CAD build for the part. Positions are in the model's coordinates, mm. A direction names the side the tool comes from. Coordinates: 2 decimals unless noted, no trailing zeros. Loops run counter-clockwise (first coordinate to the right, second up) from the corner with the lowest first, then second, coordinate; pieces in that order, holes last. Notation, with made-up numbers: (-19.5, 66) -> (21.5, 66) arc R9 ccw to (21.5, 82) -> close; hole circle Ø5 at (30, 49.5). An arc over 180 degrees is marked (long way). Answer as a JSON object with one key per item and string values. Group by question number.
from build123d import *

# Parameters (mm, degrees)
SKETCH1_W                                  = 254
SKETCH1_H                                  = 203.2
BOSS_EXTRUDE1_DEPTH                        = 6.35
SKETCH2_W                                  = 6.35
SKETCH2_H                                  = 190.5
BOSS_EXTRUDE2_DEPTH                        = 63.5
SKETCH3_W                                  = 6.35
SKETCH3_H                                  = 40.64
CUT_EXTRUDE1_DEPTH                         = 63.5
SKETCH4_W                                  = 50.8
SKETCH4_H                                  = 40.64
CUT_EXTRUDE2_DEPTH                         = 3.175
SKETCH5_W                                  = 31.75
SKETCH5_H                                  = 6.35
BOSS_EXTRUDE3_DEPTH                        = 14.912951806
SKETCH6_W                                  = 38.1
SKETCH6_H                                  = 26.67
BOSS_EXTRUDE4_DEPTH                        = 6.35
CUT_EXTRUDE3_REACH                         = 170.034
SKETCH7_R                                  = 1.85
SKETCH8_W                                  = 6.35
SKETCH8_H                                  = 50.8
CUT_EXTRUDE4_DEPTH                         = 25.4
CUT_EXTRUDE5_REACH                         = 179.004
SKETCH9_R                                  = 6.35
SKETCH10_W                                 = 40.64
SKETCH10_H                                 = 29.537048194
BOSS_EXTRUDE5_DEPTH                        = 6.35
SKETCH11_W                                 = 50.8
SKETCH11_H                                 = 12.7
BOSS_EXTRUDE6_DEPTH                        = 6.35
SKETCH12_R                                 = 1.65
CUT_EXTRUDE6_DEPTH                         = 12
MIRROR2_AT_THE_SECOND_PLANE_COPY_1_SKETC_R = 1.65
MIRROR2_AT_THE_SECOND_PLANE_COPY_1_DEPTH   = 12


with BuildPart() as part:
    # Sketch1 → Boss-Extrude1 (new body)
    with BuildSketch(Plane(origin=(0, 0, 0), x_dir=(1, 0, 0), z_dir=(0, 1, 0))):
        Rectangle(SKETCH1_W, SKETCH1_H)
    extrude(amount=BOSS_EXTRUDE1_DEPTH)

    # Sketch2 → Boss-Extrude2 (add)
    with BuildSketch(Plane(origin=(0, 6.35, 0), x_dir=(1, 0, 0), z_dir=(0, 1, 0))):
        with Locations((-123.825, 0)):
            Rectangle(SKETCH2_W, SKETCH2_H)
        Polygon((127, 101.6), (-127, 101.6), (-127, 95.25), (-120.65, 95.25), (120.65, 95.25), (127, 95.25), align=None)
        with Locations((123.825, 0)):
            Rectangle(SKETCH2_W, SKETCH2_H)
        Polygon((-120.65, -95.25), (-127, -95.25), (-127, -101.6), (127, -101.6), (127, -95.25), (120.65, -95.25), align=None)
    extrude(amount=BOSS_EXTRUDE2_DEPTH)

    # Sketch3 → Cut-Extrude1 (cut)
    with BuildSketch(Plane(origin=(0, 69.85, 0), x_dir=(1, 0, 0), z_dir=(0, 1, 0))):
        with Locations((123.825, 0)):
            Rectangle(SKETCH3_W, SKETCH3_H)
    extrude(amount=-CUT_EXTRUDE1_DEPTH, mode=Mode.SUBTRACT)

    # Sketch4 → Cut-Extrude2 (cut)
    with BuildSketch(Plane(origin=(0, 6.35, 0), x_dir=(1, 0, 0), z_dir=(0, 1, 0))):
        with Locations((101.6, 0)):
            Rectangle(SKETCH4_W, SKETCH4_H)
    extrude(amount=-CUT_EXTRUDE2_DEPTH, mode=Mode.SUBTRACT)

    # Sketch5 → Boss-Extrude3 (add)
    with BuildSketch(Plane(origin=(0, 6.35, 0), x_dir=(1, 0, 0), z_dir=(0, 1, 0))):
        with Locations((104.775, 23.495)):
            Rectangle(SKETCH5_W, SKETCH5_H)
    boss_extrude3 = extrude(amount=BOSS_EXTRUDE3_DEPTH)

    # Sketch6 → Boss-Extrude4 (add)
    with BuildSketch(Plane(origin=(0, 21.262951806, 0), x_dir=(1, 0, 0), z_dir=(0, 1, 0))):
        with Locations((107.95, 13.335)):
            Rectangle(SKETCH6_W, SKETCH6_H)
    boss_extrude4 = extrude(amount=BOSS_EXTRUDE4_DEPTH)

    # Mirror1: Boss-Extrude3, Boss-Extrude4 across plane
    add(boss_extrude3.mirror(Plane.XY))
    add(boss_extrude4.mirror(Plane.XY))

    # Sketch7 → Cut-Extrude3 (cut, up to next)
    with BuildSketch(Plane(origin=(0, 27.612951806, 0), x_dir=(1, 0, 0), z_dir=(0, 1, 0)), mode=Mode.PRIVATE) as cut_extrude3_sk1:
        with Locations(Location((99.4, 0, 0), (0, 0, 270))):
            Circle(SKETCH7_R)
    cut_extrude3_tool1 = extrude(cut_extrude3_sk1.sketch, amount=-CUT_EXTRUDE3_REACH, mode=Mode.PRIVATE) & part.part
    # Sketch7 → Cut-Extrude3 (cut, up to next)
    with BuildSketch(Plane(origin=(0, 27.612951806, 0), x_dir=(1, 0, 0), z_dir=(0, 1, 0)), mode=Mode.PRIVATE) as cut_extrude3_sk2:
        with Locations(Location((118.5, 0, 0), (0, 0, 270))):
            Circle(SKETCH7_R)
    cut_extrude3_tool2 = extrude(cut_extrude3_sk2.sketch, amount=-CUT_EXTRUDE3_REACH, mode=Mode.PRIVATE) & part.part
    add(cut_extrude3_tool1.solids().sort_by_distance((99.4, 27.612952, 0))[0], mode=Mode.SUBTRACT)
    add(cut_extrude3_tool2.solids().sort_by_distance((118.5, 27.612952, 0))[0], mode=Mode.SUBTRACT)

    # Sketch8 → Cut-Extrude4 (cut)
    with BuildSketch(Plane(origin=(0, 69.85, 0), x_dir=(1, 0, 0), z_dir=(0, 1, 0))):
        with Locations((-123.825, 50.8)):
            Rectangle(SKETCH8_W, SKETCH8_H)
    extrude(amount=-CUT_EXTRUDE4_DEPTH, mode=Mode.SUBTRACT)

    # Sketch9 → Cut-Extrude5 (cut, up to next)
    with BuildSketch(Plane.XZ, mode=Mode.PRIVATE) as cut_extrude5_sk1:
        with Locations(Location((99.4, 0, 0), (0, 0, 270))):
            Circle(SKETCH9_R)
    cut_extrude5_tool1 = extrude(cut_extrude5_sk1.sketch, amount=-CUT_EXTRUDE5_REACH, mode=Mode.PRIVATE) & part.part
    # Sketch9 → Cut-Extrude5 (cut, up to next)
    with BuildSketch(Plane.XZ, mode=Mode.PRIVATE) as cut_extrude5_sk2:
        with Locations(Location((118.5, 0, 0), (0, 0, 270))):
            Circle(SKETCH9_R)
    cut_extrude5_tool2 = extrude(cut_extrude5_sk2.sketch, amount=-CUT_EXTRUDE5_REACH, mode=Mode.PRIVATE) & part.part
    add(cut_extrude5_tool1.solids().sort_by_distance((99.4, 0, 0))[0], mode=Mode.SUBTRACT)
    add(cut_extrude5_tool2.solids().sort_by_distance((118.5, 0, 0))[0], mode=Mode.SUBTRACT)

    # Sketch10 → Boss-Extrude5 (add)
    with BuildSketch(Plane(origin=(127, 0, 0), x_dir=(0, 0, -1), z_dir=(1, 0, 0))):
        with Locations((0, 55.081475903)):
            Rectangle(SKETCH10_W, SKETCH10_H)
    extrude(amount=-BOSS_EXTRUDE5_DEPTH)

    # Sketch11 → Boss-Extrude6 (add)
    with BuildSketch(Plane.ZY.offset(127)):
        with Locations((-50.8, 63.5)):
            Rectangle(SKETCH11_W, SKETCH11_H)
    extrude(amount=-BOSS_EXTRUDE6_DEPTH)

    # Sketch12 → Cut-Extrude6 (cut)
    with BuildSketch(Plane(origin=(0, 69.85, 0), x_dir=(1, 0, 0), z_dir=(0, 1, 0))):
        with Locations(Location((-123.825, 98.425, 0), (0, 0, 270))):
            Circle(SKETCH12_R)
    cut_extrude6 = extrude(amount=-CUT_EXTRUDE6_DEPTH, mode=Mode.SUBTRACT)

    # Mirror2: Cut-Extrude6 across plane
    add(cut_extrude6.mirror(Plane.XY), mode=Mode.SUBTRACT)

    # Mirror2 at the second plane: Cut-Extrude6 across plane
    add(cut_extrude6.mirror(Plane(origin=(0, 0, 0), x_dir=(0, 0, 1), z_dir=(1, 0, 0))), mode=Mode.SUBTRACT)

    # Mirror2 at the second plane copy 1 sketc → Mirror2 at the second plane copy 1 (cut)
    with BuildSketch(Plane(origin=(0, 69.85, 0), x_dir=(-1, 0, 0), z_dir=(0, 1, 0))):
        with Locations(Location((-123.825, 98.425, 0), (0, 0, 270))):
            Circle(MIRROR2_AT_THE_SECOND_PLANE_COPY_1_SKETC_R)
    extrude(amount=-MIRROR2_AT_THE_SECOND_PLANE_COPY_1_DEPTH, mode=Mode.SUBTRACT)


solid = part.part
Item 1: Flat gauge pins, fed straight in: P1, Ø1.5, axis at x = -87, z = 9, coming from the +Y side; P2, Ø2, axis at x = 123.825, z = -98.425, coming from the +Y side. Where does each tip first touch, or does it go through?
Item 2: Band-saw the part on B-B, the plane z = -61.5. List the corners of the cut face in (x, y).
Item 3: 3-axis set-ups, long thin cutter, end or side, ignore diameter. For faces 1 (the flat face through (108, 21.263, 0)), 2 (the flat face through (88.9, 22, 0)), 3 (the flat face through (-124, 57.15, -51)): which of +Z, -Z, +X, -X, +Y, -Y reach the whole face in a straight line?
Item 4: Band-saw the part on D-D, the plane z = 75. List the corners of the cut face in (x, y).
Item 5: Band-saw the part on A-A, the plane z = 15. List the corners of the cut face in (x, y) (3 decimals).
Item 6: Pull direction Y, two halves, no side cores. Call faces 4 (the flat face through (-1, 69.85, -98)), 5 (the flat face through (124, 34, 20.32)), 6 (the flat face through (-2, 34, 101.6)): +Y half, -Y half, draft (parallel to the pull), parting line (faces both ways), or undercut.
Item 7: Drill centre lines: L1, parallel to X at y = 25.75, z = 0; L2, parallel to X at y = 50, z = 56; L3, parallel to Z at x = -75.5, y = 54. Where is each one in solid material? Low to high.
Item 8: Band-saw the part on C-C, the plane x = -55.5. List the corners of the cut face in (y, z), and give its area (3 significant figures).
Reply:
{
 "1": {"P1": "y = 6.35", "P2": "y = 57.85"},
 "2": {"outline": "(-127, 0) -> (127, 0) -> (127, 69.85) -> (120.65, 69.85) -> (120.65, 6.35) -> (-120.65, 6.35) -> (-120.65, 44.45) -> (-127, 44.45) -> close; (-127, 57.15) -> (-120.65, 57.15) -> (-120.65, 69.85) -> (-127, 69.85) -> close"},
 "3": {"face 1": "+X", "face 2": "+Y", "face 3": "-X"},
 "4": {"outline": "(-127, 0) -> (127, 0) -> (127, 69.85) -> (120.65, 69.85) -> (120.65, 6.35) -> (-120.65, 6.35) -> (-120.65, 69.85) -> (-127, 69.85) -> close"},
 "5": {"outline": "(-127, 0) -> (127, 0) -> (127, 3.175) -> (76.2, 3.175) -> (76.2, 6.35) -> (-120.65, 6.35) -> (-120.65, 69.85) -> (-127, 69.85) -> close; (88.9, 21.263) -> (127, 21.263) -> (127, 27.613) -> (88.9, 27.613) -> close; (120.65, 40.313) -> (127, 40.313) -> (127, 69.85) -> (120.65, 69.85) -> close"},
 "6": {"face 4": "+Y half", "face 5": "undercut", "face 6": "draft"},
 "7": {"L1": "-127 to -120.65, 88.9 to 97.55, 101.25 to 116.65, 120.35 to 127", "L2": "-127 to -120.65, 120.65 to 127", "L3": "-101.6 to -95.25, 95.25 to 101.6"},
 "8": {"outline": "(0, -101.6) -> (69.85, -101.6) -> (69.85, -95.25) -> (6.35, -95.25) -> (6.35, 95.25) -> (69.85, 95.25) -> (69.85, 101.6) -> (0, 101.6) -> close", "area": "2,100 mm²"}
}
